from build123d import *

# Parameters (mm, degrees)
SKETCH1_W                   = 30.95625
SKETCH1_H                   = 88.9
BOSS_EXTRUDE1_DEPTH         = 4.7625
FILLET1_R                   = 2.54
SKETCH6_R                   = 1.524
CUT_EXTRUDE1_DEPTH          = 5.7625
SKETCH7_R                   = 2.38125
CUT_EXTRUDE2_DEPTH          = 5.7625
BOSS_EXTRUDE3_DEPTH         = 1.524
F_4_40_TAPPED_HOLE1_D       = 2.2606
SKETCH10_R                  = 1.524
CUT_EXTRUDE3_DEPTH          = 2.524
SKETCH11_R                  = 3.175
CUT_EXTRUDE4_DEPTH          = 3.302
F_1_2_13_TAPPED_HOLE2_D     = 10.71626
F_1_2_13_TAPPED_HOLE2_DEPTH = 2.794
F_1_2_13_TAPPED_HOLE2_TIP   = 3.219489309


with BuildPart() as part:
    # Sketch1 → Boss-Extrude1 (new body)
    with BuildSketch(Plane(origin=(0, 0, 0), x_dir=(1, 0, 0), z_dir=(0, 1, 0))):
        Rectangle(SKETCH1_W, SKETCH1_H)
    extrude(amount=BOSS_EXTRUDE1_DEPTH)

    # Fillet1
    fillet1_edges = [part.edges().sort_by_distance(p)[0] for p in [
        (15.478125, 2.38125, -44.45),
        (15.478125, 2.38125, 44.45),
        (-15.478125, 2.38125, 44.45),
        (-15.478125, 2.38125, -44.45),
    ]]
    fillet(fillet1_edges, radius=FILLET1_R)

    # Sketch6 → Cut-Extrude1 (cut, through all)
    with BuildSketch(Plane.XZ):
        with Locations((0, 14.478)):
            Circle(SKETCH6_R)
        with Locations((0, -14.478)):
            Circle(SKETCH6_R)
    extrude(amount=-CUT_EXTRUDE1_DEPTH, mode=Mode.SUBTRACT)

    # Sketch7 → Cut-Extrude2 (cut, through all)
    with BuildSketch(Plane.XZ):
        with Locations((0, -39.116)):
            Circle(SKETCH7_R)
        with Locations((0, 39.116)):
            Circle(SKETCH7_R)
    extrude(amount=-CUT_EXTRUDE2_DEPTH, mode=Mode.SUBTRACT)

    # Sketch9 → Boss-Extrude3 (add)
    with BuildSketch(Plane.XZ):
        with BuildLine():
            Line((12.938125, -44.45), (-12.938125, -44.45))
            ThreePointArc((-12.938125, -44.45), (-14.734176224, -43.706051224), (-15.478125, -41.91))
            Line((-15.478125, -41.91), (-15.478125, 41.91))
            ThreePointArc((-15.478125, 41.91), (-14.734176224, 43.706051224), (-12.938125, 44.45))
            Line((-12.938125, 44.45), (12.938125, 44.45))
            ThreePointArc((12.938125, 44.45), (14.734176224, 43.706051224), (15.478125, 41.91))
            Line((15.478125, 41.91), (15.478125, -41.91))
            ThreePointArc((15.478125, -41.91), (14.734176224, -43.706051224), (12.938125, -44.45))
        make_face()
    extrude(amount=BOSS_EXTRUDE3_DEPTH)

    # #4-40 Tapped Hole1 (through all)
    with Locations(Plane(origin=(0, 4.7625, 0), x_dir=(-1, 0, 0), z_dir=(0, 1, 0))):
        with Locations((0, 25.4), (0, -25.4)):
            Hole(F_4_40_TAPPED_HOLE1_D / 2)

    # Sketch10 → Cut-Extrude3 (cut, through all)
    with BuildSketch(Plane(origin=(0, 0, 0), x_dir=(1, 0, 0), z_dir=(0, 1, 0))):
        with Locations((0, -14.478)):
            Circle(SKETCH10_R)
        with Locations((0, 14.478)):
            Circle(SKETCH10_R)
    extrude(amount=-CUT_EXTRUDE3_DEPTH, mode=Mode.SUBTRACT)

    # Sketch11 → Cut-Extrude4 (cut)
    with BuildSketch(Plane.XZ.offset(1.524)):
        with Locations((0, -14.478)):
            Circle(SKETCH11_R)
        with Locations((0, 14.478)):
            Circle(SKETCH11_R)
    extrude(amount=-CUT_EXTRUDE4_DEPTH, mode=Mode.SUBTRACT)

    # 1/2-13 Tapped Hole2
    with Locations(Plane(origin=(0, 4.7625, 0), x_dir=(-1, 0, 0), z_dir=(0, 1, 0))):
        with Locations((0, 0)):
            Hole(F_1_2_13_TAPPED_HOLE2_D / 2, depth=F_1_2_13_TAPPED_HOLE2_DEPTH)
            with Locations((0, 0, -(F_1_2_13_TAPPED_HOLE2_DEPTH + F_1_2_13_TAPPED_HOLE2_TIP / 2))):  # 118° drill point
                Cone(0, F_1_2_13_TAPPED_HOLE2_D / 2, F_1_2_13_TAPPED_HOLE2_TIP, mode=Mode.SUBTRACT)


solid = part.part
The model under review builds one solid part; all positions refer to its coordinate system, in mm. A direction names the side the tool comes from. Round coordinates to 2 decimals unless told otherwise and drop trailing zeros. Loops run counter-clockwise (first coordinate to the right, second up) from the corner with the lowest first, then second, coordinate; pieces in that order, holes last. Notation, with made-up numbers: (19.5, 10.5) - (23.5, 10.5) arc R12 cw to (23.5, 22.5) - close; hole circle Ø9 at (87.5, 21.5). An arc over 180 degrees is marked (long way). Use CSV: the item, a comma, the result in double quotes.
(1) The part is to be moulded in two halves that separate along X. For faces 4 (the flat face through (15.478, 2, 1)), 5 (the flat face through (-7, 4.762, -1)), 6 (the flat face through (0, 0, 39)), 7 (the flat face through (-15.478, 2, -1)), say which applies: pulls with the +X half, pulls with the -X half, needs draft (parallel to the pull), parting line crosses it, or undercut.
Working result:
face 4,"pulls with the +X half"
face 5,"needs draft"
face 6,"undercut"
face 7,"pulls with the -X half"
(2) Take a section at A-A, the plane z = 25.4. Give the boundary of the cut face in (x, y), plus the area to 3 significant figures.
Working result:
outline,"(-15.48, -1.52) - (-1.13, -1.52) - (-1.13, 4.76) - (-15.48, 4.76) - close; (1.13, -1.52) - (15.48, -1.52) - (15.48, 4.76) - (1.13, 4.76) - close"
area,"180 mm^2"
(3) Take a section at B-B, the plane y = 1. State how many separate pieces and enclosed holes the cut face has, plus the area to 3 significant figures.
Working result:
separate pieces,"1"
enclosed holes,"7"
area,"2,600 mm^2"
(4) Machinability: for faces 1 (the flat face through (0, 2, -44.45)), 2 (the cylindrical face through (-0.688, 0.104, -17.577)), 3 (the cylindrical face through (2.472, 3.346, -4.754)), which of the approach directions +Z, -Z, +X, -X, +Y, -Y give a long, thin tool a straight path to every point of the face, cutting with its end or side? Answer none if there is none.
Working result:
face 1,"-Z, +X, -X, +Y, -Y"
face 2,"-Y"
face 3,"+Y"
(5) For line 1 (X direction, y = 3, z = -14.5); line 2 (Z direction, x = 0, y = -0.75); line 3 (X direction, y = 1.5, z = 2.5), list the stretches that pass through material, from the lowest coordinate up.
Working result:
line 1,"x = -15.48 to -1.52, 1.52 to 15.48"
line 2,"z = -44.45 to -26.53, -24.27 to -17.65, -11.3 to -0.83, 0.83 to 11.3, 17.65 to 24.27, 26.53 to 44.45"
line 3,"x = -15.48 to -3.84, 3.84 to 15.48"
(6) Clearance check with flat-ended pins moving along their axes: P1, Ø4.5, axis at x = 0, z = 39.116, coming from the +Y side; P2, Ø5, axis at x = 0, z = 14.478, coming from the -Y side. State where each tip first meets the part, or that it passes through.
Working result:
P1,"stops at y = 0"
P2,"stops at y = 1.78"
